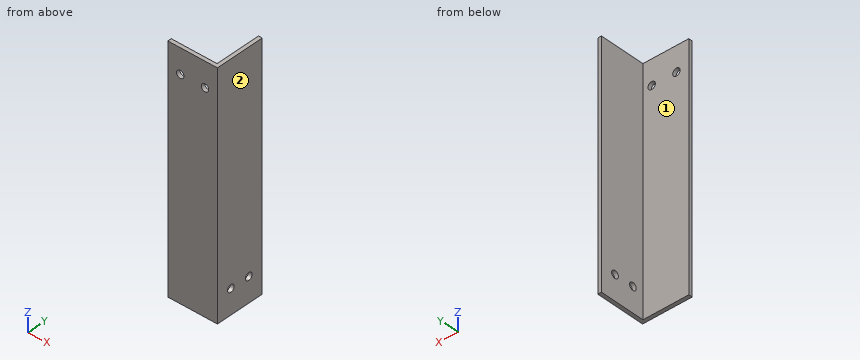
from build123d import *

# Parameters (mm, degrees)
EXTRUSION1_DEPTH = 96
ESQUISSE2_R      = 1.5
EXTRUSION2_DEPTH = 70
ESQUISSE3_R      = 1.5
EXTRUSION3_DEPTH = 10


with BuildPart() as part:
    # Esquisse1 → Extrusion1 (new body)
    with BuildSketch(Plane.XY):
        Polygon((-3.718958969, 18.5), (-3.718958969, -1.5), (-23.718958969, -1.5), (-23.718958969, 0), (-5.218958969, 0), (-5.218958969, 18.5), align=None)
    extrude(amount=EXTRUSION1_DEPTH)

    # Esquisse2 → Extrusion2 (cut)
    with BuildSketch(Plane.XZ.offset(1.5)):
        with Locations((-8.718958969, 86)):
            Circle(ESQUISSE2_R)
        with Locations((-18.718958969, 86)):
            Circle(ESQUISSE2_R)
    extrude(amount=-EXTRUSION2_DEPTH, mode=Mode.SUBTRACT)

    # Esquisse3 → Extrusion3 (cut)
    with BuildSketch(Plane(origin=(-3.718958969, 0, 0), x_dir=(0, 0, -1), z_dir=(1, 0, 0))):
        with Locations(Location((-10, 12.5, 0), (0, 0, 90))):
            Circle(ESQUISSE3_R)
        with Locations(Location((-10, 4.5, 0), (0, 0, 90))):
            Circle(ESQUISSE3_R)
    extrude(amount=-EXTRUSION3_DEPTH, mode=Mode.SUBTRACT)


solid = part.part
Work out the finished part from the listing and answer in its coordinate system (mm). Face numbers are marked on the shaded views. A direction names the side the tool comes from. Round coordinates to 2 decimals unless told otherwise and drop trailing zeros. Write each loop counter-clockwise with the first axis right and the second up, starting at its lowest first coordinate (ties: lowest second). Pieces come first, ordered by that corner, then holes. Notation, with made-up numbers: (-22, 38.5) - (37, 38.5) arc R18 ccw to (37, 70.5) - close; hole circle Ø3 at (77.25, 55.5). An arc over 180 degrees is marked (long way). Answer in a Markdown table with one row per item. Add a question column.
1. A cutting plane is placed at D-D, the plane z = 48. Determine the outline of the cut face in (x, y).
2. A cutting plane is placed at B-B, the plane y = 12.5. Determine the outline of the cut face in (x, z).
3. Given pin 1 (4 mm diameter, centred on y = 4.5, z = 10, fed in from -X); pin 2 (1.8 mm diameter, centred on x = -8.72, z = 86, fed in from -Y); pin 3 (3 mm diameter, centred on x = -18, z = 19, fed in from +Y), each flat-ended and moving along its own axis, determine where each tip first touches the part or whether it passes through.
4. For the marked faces 1 and 2, determine the directions among +Z, -Z, +X, -X, +Y, -Y from which every point of the face is accessible in a straight line to the end or side of a thin tool.
5. A cutting plane is placed at A-A, the plane z = 10. Determine the outline of the cut face in (x, y).
6. A cutting plane is placed at C-C, the plane x = -9. Determine the outline of the cut face in (y, z).
7. Find the intervals of material crossed by line 1 along X through (y, z) = (-1.2, 86); line 2 along Z through (x, y) = (-4.3, 12.5); line 3 along X through (y, z) = (2.25, 37.5), in increasing order. Write a range as from..to.
Worked out:
| question | item | result |
|---|---|---|
| 1 | outline | (-23.72, -1.5) - (-3.72, -1.5) - (-3.72, 18.5) - (-5.22, 18.5) - (-5.22, 0) - (-23.72, 0) - close |
| 2 | outline | (-5.22, 0) - (-3.72, 0) - (-3.72, 8.5) - (-5.22, 8.5) - close; (-5.22, 11.5) - (-3.72, 11.5) - (-3.72, 96) - (-5.22, 96) - close |
| 3 | pin 1 | x = -5.22 |
| 3 | pin 2 | through |
| 3 | pin 3 | y = 0 |
| 4 | face 1 | +Z, -Z, -X, +Y |
| 4 | face 2 | +Z, -Z, +X, +Y, -Y |
| 5 | outline | (-23.72, -1.5) - (-3.72, -1.5) - (-3.72, 3) - (-5.22, 3) - (-5.22, 0) - (-23.72, 0) - close; (-5.22, 6) - (-3.72, 6) - (-3.72, 11) - (-5.22, 11) - close; (-5.22, 14) - (-3.72, 14) - (-3.72, 18.5) - (-5.22, 18.5) - close |
| 6 | outline | (-1.5, 0) - (0, 0) - (0, 84.53) - (-1.5, 84.53) - close; (-1.5, 87.47) - (0, 87.47) - (0, 96) - (-1.5, 96) - close |
| 7 | line 1 | -23.72..-20.22, -17.22..-10.22, -7.22..-3.72 |
| 7 | line 2 | 0..8.5, 11.5..96 |
| 7 | line 3 | -5.22..-3.72 |
